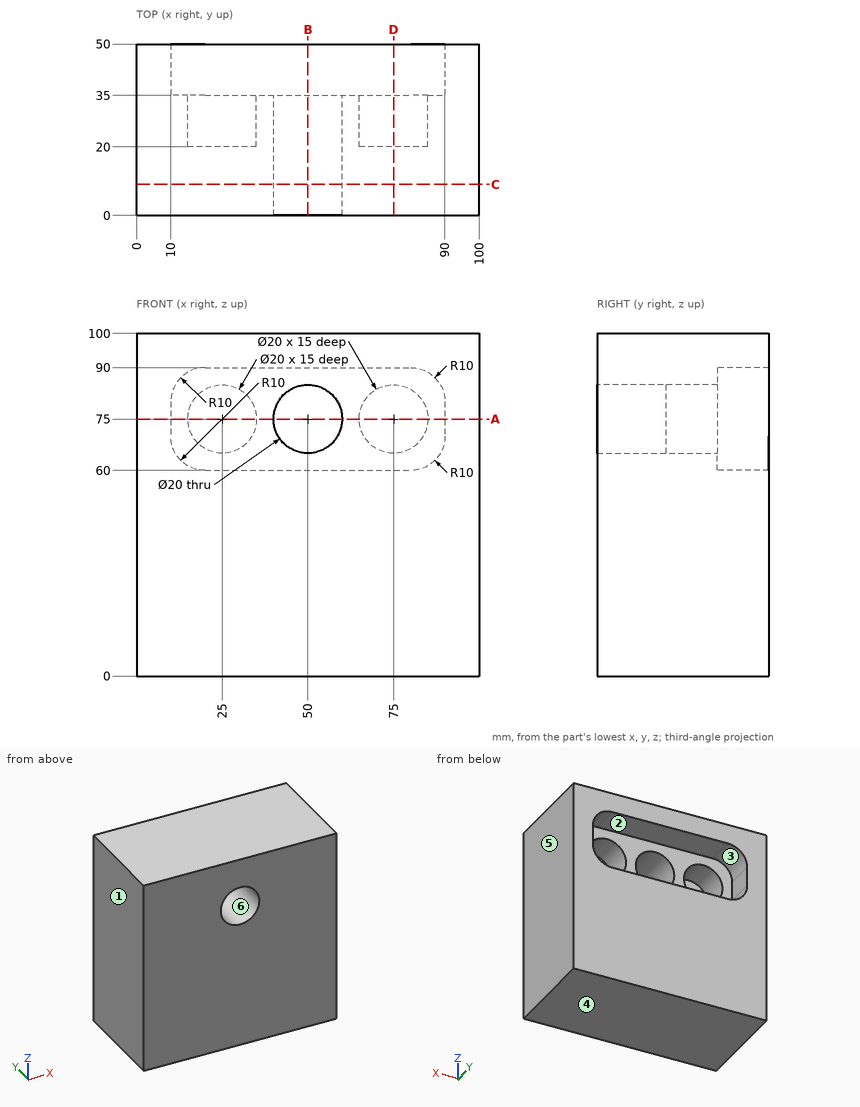
Can you work these out from the drawing? Everything is in mm from the part's minimum corner. A direction names the side the tool comes from. Round coordinates to 2 decimals unless told otherwise and drop trailing zeros. Loops run counter-clockwise (first coordinate to the right, second up) from the corner with the lowest first, then second, coordinate; pieces in that order, holes last. Notation, with made-up numbers: (14, 39) - (41, 39) arc R15 ccw to (41, 55) - close; hole circle Ø7 at (51.5, 8). An arc over 180 degrees is marked (long way). Answer in a Markdown table with one row per item. Add a question column.
Q1. I want a section at C-C on y = 9. List the corners of the cut face in (x, z) for me.
Q2. For pin 1 Ø12 at (x, z) = (45.5, 63.5) entering from +Y; pin 2 Ø18 at (x, z) = (25, 75) entering from +Y; pin 3 Ø15 at (x, z) = (66.5, 79.5) entering from +Y, each with a flat end and sliding along its axis, tell me the tip position at first contact or that it passes through.
Q3. I need wall thicknesses on L1, parallel to X at y = 28, z = 75; L2, parallel to X at y = 10, z = 75; L3, parallel to Z at x = 24.5, y = 32.5. Which ranges of each line are inside material? Lowest first, please.
Q4. We'd pull the mould along X, two halves only. Please class the marked faces 3, 4, 5 and 6: pulls with the +X half, pulls with the -X half, needs draft (parallel to the pull), parting line crosses it, or undercut.
Q5. I want a section at D-D on x = 75. List the corners of the cut face in (y, z) for me.
Q6. I want a section at A-A on z = 75. List the corners of the cut face in (x, y) for me.
Q7. Which directions (+Z, -Z, +X, -X, +Y, -Y) give clear straight access to the entire face, cutting with the end or side of a thin tool? Please do the marked faces 1 and 2.
Q8. I want a section at B-B on x = 50. List the corners of the cut face in (y, z) for me.
A:
| question | item | result |
|---|---|---|
| 1 | outline | (0, 0) - (100, 0) - (100, 100) - (0, 100) - close; hole circle Ø20 at (50, 75) |
| 2 | pin 1 | y = 50 |
| 2 | pin 2 | y = 20 |
| 2 | pin 3 | y = 35 |
| 3 | L1 | 0 to 15, 35 to 40, 60 to 65, 85 to 100 |
| 3 | L2 | 0 to 40, 60 to 100 |
| 3 | L3 | 0 to 65.01, 84.99 to 100 |
| 4 | face 3 | undercut |
| 4 | face 4 | needs draft |
| 4 | face 5 | pulls with the +X half |
| 4 | face 6 | undercut |
| 5 | outline | (0, 0) - (50, 0) - (50, 60) - (35, 60) - (35, 65) - (20, 65) - (20, 85) - (35, 85) - (35, 90) - (50, 90) - (50, 100) - (0, 100) - close |
| 6 | outline | (0, 0) - (40, 0) - (40, 35) - (35, 35) - (35, 20) - (15, 20) - (15, 35) - (10, 35) - (10, 50) - (0, 50) - close; (60, 0) - (100, 0) - (100, 50) - (90, 50) - (90, 35) - (85, 35) - (85, 20) - (65, 20) - (65, 35) - (60, 35) - close |
| 7 | face 1 | +Z, -Z, -X, +Y, -Y |
| 7 | face 2 | +Y |
| 8 | outline | (0, 0) - (50, 0) - (50, 60) - (35, 60) - (35, 65) - (0, 65) - close; (0, 85) - (35, 85) - (35, 90) - (50, 90) - (50, 100) - (0, 100) - close |
